```python
from build123d import *

# Parameters (mm, degrees)
F0_R     = 57
F0_R_2   = 54.5
F0_R_3   = 15
F0_R_4   = 13
F1_DEPTH = 3
F2_DEPTH = 5
F3_DEPTH = 10


with BuildPart() as f1:
    # F0 (on Top) → F1 (new body)
    with BuildSketch(Plane.XY):
        Circle(F0_R)
        Circle(F0_R_2, mode=Mode.SUBTRACT)
        Circle(F0_R_2)
        Circle(F0_R_3, mode=Mode.SUBTRACT)
        Circle(F0_R_3)
        Circle(F0_R_4, mode=Mode.SUBTRACT)
    extrude(amount=-F1_DEPTH)

    # F0 (on Top) → F2 (join)
    with BuildSketch(Plane.XY):
        Circle(F0_R)
        Circle(F0_R_2, mode=Mode.SUBTRACT)
    extrude(amount=F2_DEPTH)

    # F0 (on Top) → F3 (join)
    with BuildSketch(Plane.XY):
        Circle(F0_R_3)
        Circle(F0_R_4, mode=Mode.SUBTRACT)
    extrude(amount=F3_DEPTH)


solid = f1.part
```
For this review, take the finished solid that the model builds, in its own axes (mm). A direction names the side the tool comes from. Coordinates: 2 decimals unless noted, no trailing zeros. Order: outer loops, then holes, each group sorted by start corner. A loop starts at its lowest first (then second) coordinate and runs counter-clockwise, first axis right, second up. Notation, with made-up numbers: (74.5, 13) -> (130.5, 13) arc R23 cw to (130.5, 38) -> close; hole circle Ø4 at (40.25, -4). An arc over 180 degrees is marked (long way). Use CSV: the item, a comma, the result in double quotes. Start each with the question number.
Item 1: We need section C-C, the plane z = 2.75. Give the boundary of the cut face in (x, y).
Item 2: Insertion check: pin 1 (1.5 mm diameter, centred on y = -18.5, z = 0.5, fed in from +X); pin 2 (8 mm diameter, centred on x = -32.5, y = -32, fed in from +Z); pin 3 (4 mm diameter, centred on x = 35.5, z = -0.5, fed in from -Y); pin 4 (3 mm diameter, centred on x = 10, y = 5.5, fed in from -Z). Each pin has a flat end and moves straight along its axis. Give the tip position at first contact, or say it passes through.
Item 3: We need section A-A, the plane x = 0. Give the boundary of the cut face in (y, z).
Item 4: We need section D-D, the plane x = 41. Give the boundary of the cut face in (y, z).
Item 5: For faces 5 (the face through (-43.25, -33.16, 2.46)), 6 (the face through (-10.316, -7.91, 3.409)), list the 3-axis set-ups (+Z, -Z, +X, -X, +Y, -Y) from which the entire face can be reached by the end or side of a thin tool; tool diameter is ignored.
Item 6: Wall thickness on probe 1 along Y at (x, z) = (0, 3.5); probe 2 along Y at (x, z) = (0, 6); probe 3 along Z at (x, y) = (-15.5, -36): over which ranges is each line inside the solid? List them lowest first.
Item 7: Draft analysis for pull direction Y (two halves, no side actions). For faces 1 (the face through (46.2, -29.3, 5)), 2 (the face through (52.654, -21.831, 1.056)), 3 (the face through (11, -11, 0)), 4 (the face through (-14.985, 0.66, 4.93)), state which applies: pulls with the +Y half, pulls with the -Y half, needs draft (parallel to the pull), parting line crosses it, or undercut.
Derived:
1,outline,"circle Ø114 at (0, 0); circle Ø30 at (0, 0); hole circle Ø109 at (0, 0); hole circle Ø26 at (0, 0)"
2,pin 1,"stops at x = 54.17"
2,pin 2,"stops at z = 0"
2,pin 3,"stops at y = -46.12"
2,pin 4,"passes through"
3,outline,"(-57, -3) -> (-13, -3) -> (-13, 10) -> (-15, 10) -> (-15, 0) -> (-54.5, 0) -> (-54.5, 5) -> (-57, 5) -> close; (13, -3) -> (57, -3) -> (57, 5) -> (54.5, 5) -> (54.5, 0) -> (15, 0) -> (15, 10) -> (13, 10) -> close"
4,outline,"(-39.6, -3) -> (39.6, -3) -> (39.6, 5) -> (35.91, 5) -> (35.91, 0) -> (-35.91, 0) -> (-35.91, 5) -> (-39.6, 5) -> close"
5,face 5,"+Z"
5,face 6,"+Z, -Z"
6,probe 1,"y = -57 to -54.5, -15 to -13, 13 to 15, 54.5 to 57"
6,probe 2,"y = -15 to -13, 13 to 15"
6,probe 3,"z = -3 to 0"
7,face 1,"needs draft"
7,face 2,"parting line crosses it"
7,face 3,"undercut"
7,face 4,"undercut"
